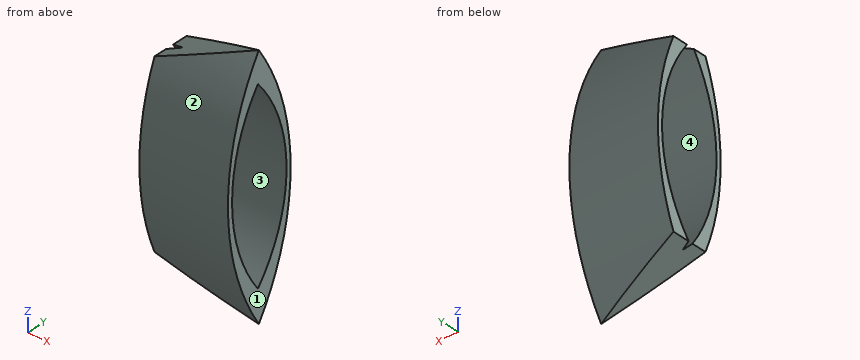
from build123d import *

# Parameters (mm, degrees)
F0_W     = 50
F0_H     = 140
F1_DEPTH = 42
F3_DEPTH = 42
F5_DEPTH = 50
F7_DEPTH = 50
F9_DEPTH = 50


with BuildPart() as f1:
    # F0 (on Front) → F1 (new body)
    with BuildSketch(Plane.XZ):
        Rectangle(F0_W, F0_H)
    extrude(amount=F1_DEPTH)

    # F2 (on face) → F3 (cut)
    with BuildSketch(Plane.XZ.offset(42)):
        Polygon((25, 70), (-25, 70), (-25, 50), align=None)
        Polygon((-25, -50), (-25, -70), (25, -70), align=None)
    extrude(amount=-F3_DEPTH, mode=Mode.SUBTRACT)

    # F4 (on face) → F5 (cut)
    with BuildSketch(Plane.YZ.offset(25)):
        with BuildLine():
            ThreePointArc((-21, -70), (-40.967372, 0), (-21, 70))
            Line((-21, 70), (-47.731567, 70))
            Line((-47.731567, 70), (-47.731567, -70))
            Line((-47.731567, -70), (-21, -70))
        make_face()
    extrude(amount=-F5_DEPTH, mode=Mode.SUBTRACT)

    # F6 (on face) → F7 (cut)
    with BuildSketch(Plane.YZ.offset(25)):
        with BuildLine():
            ThreePointArc((-21, 70), (-0.464572, 0), (-21, -70))
            Line((-21, -70), (3.54092, -70))
            Line((3.54092, -70), (3.54092, 70))
            Line((3.54092, 70), (-21, 70))
        make_face()
    extrude(amount=-F7_DEPTH, mode=Mode.SUBTRACT)

    # F8 (on face) → F9 (cut)
    with BuildSketch(Plane.YZ.offset(25)):
        with BuildLine():
            ThreePointArc((-21.610456, 53.072974), (-38.307918, 0.665912), (-21.610456, -51.741149))
            ThreePointArc((-21.610456, -51.741149), (-3.101031, 0.665912), (-21.610456, 53.072974))
        make_face()
    extrude(amount=-F9_DEPTH, mode=Mode.SUBTRACT)


solid = f1.part
CAD build for the part. Positions are in the model's coordinates, mm. Face numbers are marked on the shaded views. Coordinates: 2 decimals unless noted, no trailing zeros. Loops run counter-clockwise (first coordinate to the right, second up) from the corner with the lowest first, then second, coordinate; pieces in that order, holes last. Notation, with made-up numbers: (-14, 39) - (15, 39) arc R29 ccw to (15, 71) - close; hole circle Ø2 at (18, 37.5). An arc over 180 degrees is marked (long way). Use one line per item in the form item = value. Start each with the question number.
1) Band-saw the part on D-D (y = -17.5). Give the cut face in (x, z).
2) Two-plate mould, pull along Y, no slides. Class the marked faces 1, 2, 3 and 4: +Y half, -Y half, draft (parallel to the pull), parting line (faces both ways), or undercut.
3) Band-saw the part on B-B (y = -5). Give the cut face in (x, z), and give its area (3 significant figures).
4) Drill centre lines: L1, parallel to Y at x = -8, z = 5; L2, parallel to Z at x = 0.5, y = -21; L3, parallel to Y at x = -8, z = 20. Where is each one in solid material? Low to high. Write a range as from..to.
5) Band-saw the part on C-C (x = -0.5). Give the cut face in (y, z), and give its area (3 significant figures).
6) Band-saw the part on A-A (z = 1). Give the cut face in (x, y), and give its area (3 significant figures).
7) Flat gauge pins, fed straight in: pin 1 (4 mm diameter, centred on x = 7.5, y = -17, fed in from +Z); pin 2 (10 mm diameter, centred on x = 4, y = -36, fed in from -Z); pin 3 (1 mm diameter, centred on x = 12.5, y = -25.5, fed in from -Z). Where does each tip first touch, or does it go through?
Check values:
q1.outline = (-25, -50) - (10.56, -64.22) - (25, -64.22) - (25, -46.19) - (-25, -46.19) - close; (-25, 47.52) - (25, 47.52) - (25, 64.22) - (10.56, 64.22) - (-25, 50) - close
q2.face_1 = draft
q2.face_2 = -Y half
q2.face_3 = undercut
q2.face_4 = undercut
q3.outline = (-25, -33.98) - (25, -33.98) - (25, -17.03) - (-25, -17.03) - close; (-25, 18.37) - (25, 18.37) - (25, 33.98) - (-25, 33.98) - close
q3.area = 1,630 mm2
q4.L1 = -40.87..-38.2, -3.21..-0.56
q4.L2 = -60.2..-50.98, 52.31..60.2
q4.L3 = -39.45..-36.22, -5.37..-2.02
q5.outline = (-26.73, -59.8) - (-15.09, -59.8) arc R129.57 ccw to (-15.09, 59.8) - (-26.73, 59.8) arc R132.68 ccw to start; hole (-21.61, -51.74) arc R83.45 ccw to (-21.61, 53.07) arc R90.59 ccw to start
q5.area = 1,200 mm2
q6.outline = (-25, -40.96) - (25, -40.96) - (25, -38.31) - (-25, -38.31) - close; (-25, -3.1) - (25, -3.1) - (25, -0.47) - (-25, -0.47) - close
q6.area = 264 mm2
q7.pin_1 = 63.79
q7.pin_2 = -50.45
q7.pin_3 = -63.11
